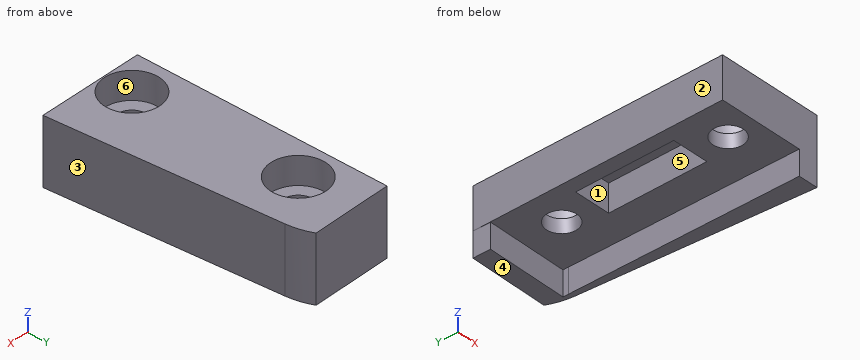
```python
from build123d import *

# Parameters (mm, degrees)
BOSS_EXTRUDE1_DEPTH = 1.8
SKETCH3_R           = 1.1
BOSS_EXTRUDE2_DEPTH = 3
SKETCH4_W           = 2.663520563
SKETCH4_H           = 7.169309516
CUT_EXTRUDE1_DEPTH  = 2
SKETCH5_R           = 2
CUT_EXTRUDE2_DEPTH  = 2


with BuildPart() as part:
    # Sketch1 → Boss-Extrude1 (new body)
    with BuildSketch(Plane(origin=(0, 0, 0), x_dir=(0, 1, 0), z_dir=(0, 0, 1))):
        with BuildLine():
            Line((6.830014349, -2.344806069), (-9.690684049, -3.631823148))
            Line((-9.690684049, -3.631823148), (-9.690684049, -2.205416312))
            Line((-9.690684049, -2.205416312), (6.947514193, -1.975901922))
            Line((6.947514193, -1.975901922), (7.350857331, -1.970338035))
            Line((7.350857331, -1.970338035), (7.269057374, 3.9595904))
            Line((7.269057374, 3.9595904), (8.531793523, 3.982646507))
            Line((8.531793523, 3.982646507), (8.638213972, -1.845785322))
            ThreePointArc((8.638213972, -1.845785322), (7.758081535, -2.182141378), (6.830014349, -2.344806069))
        make_face()
    extrude(amount=BOSS_EXTRUDE1_DEPTH)

    # Sketch3 → Boss-Extrude2 (add)
    with BuildSketch(Plane.XY.offset(1.8)):
        with BuildLine():
            Line((-3.982646507, 8.531793523), (-3.982646507, -9.690684049))
            Line((-3.982646507, -9.690684049), (3.631823148, -9.690684049))
            Line((3.631823148, -9.690684049), (2.344806069, 6.830014349))
            ThreePointArc((2.344806069, 6.830014349), (2.182141378, 7.758081535), (1.845785322, 8.638213972))
            Line((1.845785322, 8.638213972), (-3.982646507, 8.531793523))
        make_face()
        with Locations((-1.223821134, -7.594621825)):
            Circle(SKETCH3_R, mode=Mode.SUBTRACT)
        with Locations((-1.389338495, 4.404236621)):
            Circle(SKETCH3_R, mode=Mode.SUBTRACT)
    extrude(amount=BOSS_EXTRUDE2_DEPTH)

    # Sketch4 → Cut-Extrude1 (cut)
    with BuildSketch(Plane(origin=(0, 0, 1.8), x_dir=(1, 0, 0), z_dir=(0, 0, -1))):
        with Locations((-1.621806935, 1.615257833)):
            Rectangle(SKETCH4_W, SKETCH4_H)
    extrude(amount=-CUT_EXTRUDE1_DEPTH, mode=Mode.SUBTRACT)

    # Sketch5 → Cut-Extrude2 (cut)
    with BuildSketch(Plane.XY.offset(4.8)):
        with Locations((-1.389338495, 4.404236621)):
            Circle(SKETCH5_R)
        with Locations((-1.223821134, -7.594621825)):
            Circle(SKETCH5_R)
    extrude(amount=-CUT_EXTRUDE2_DEPTH, mode=Mode.SUBTRACT)


solid = part.part
```
Can you work these out from the model? Positions are in its coordinate system, mm. Face numbers are marked on the shaded views. A direction names the side the tool comes from. Give positions to 0.01 mm unless a question says otherwise; leave off trailing zeros. Loops run counter-clockwise (first coordinate to the right, second up) from the corner with the lowest first, then second, coordinate; pieces in that order, holes last. Notation, with made-up numbers: M 1.25,62 L 14.25,62 A24 cw 14.25,83 Z; hole C -7,51.25 d7. An arc over 180 degrees is marked long. Answer in a Markdown table with one row per item.
1. Which directions (+Z, -Z, +X, -X, +Y, -Y) give clear straight access to the entire face, cutting with the end or side of a thin tool? Please do the marked faces 4, 5 and 6.
Taken from the geometry:
| item | result |
|---|---|
| face 4 | -Z, +X, -X, +Y, -Y |
| face 5 | -Z |
| face 6 | +Z |
2. Thinking about a two-plate mould opening in X: for the marked faces 1, 2 and 3, which applies, released by +X, released by -X, zero draft, split by the parting line, or undercut?
Taken from the geometry:
| item | result |
|---|---|
| face 1 | undercut |
| face 2 | released by -X |
| face 3 | released by +X |
3. Suppose I cut it at A-A on z = 2.15. Write out the boundary of the cut face in (x, y), plus the area to 3 significant figures.
Taken from the geometry:
| item | result |
|---|---|
| outline | M -3.98,-9.69 L 3.63,-9.69 L 2.34,6.83 A4.93 ccw 1.85,8.64 L -3.98,8.53 Z; hole M -2.95,-5.2 L -0.29,-5.2 L -0.29,1.97 L -2.95,1.97 Z; hole C -1.39,4.4 d2.2; hole C -1.22,-7.59 d2.2 |
| area | 99.3 mm² |
4. For pin 1 Ø1.6 at (x, z) = (-1.5, 3) entering from +Y; pin 2 Ø1.2 at (x, y) = (-1.5, 5) entering from +Z; pin 3 Ø2 at (x, y) = (-2, -0.5) entering from -Z, each with a flat end and sliding along its axis, tell me the tip position at first contact or that it passes through.
Taken from the geometry:
| item | result |
|---|---|
| pin 1 | stops at y = 8.59 |
| pin 2 | stops at z = 2.8 |
| pin 3 | stops at z = 1.8 |
5. If I drill on line 1 along X through (y, z) = (1, 2.95); line 2 along Y through (x, z) = (-1.5, 2.2); line 3 along Y through (x, z) = (-1, 1.9), over which ranges is the centre line in solid material (lowest first)?
Taken from the geometry:
| item | result |
|---|---|
| line 1 | x = -3.98 to -2.95, -0.29 to 2.8 |
| line 2 | y = -9.69 to -8.66, -6.53 to -5.2, 1.97 to 3.31, 5.5 to 8.58 |
| line 3 | y = -9.69 to -8.67, -6.52 to -5.2, 1.97 to 3.38, 5.43 to 8.59 |
6. Suppose I cut it at C-C on z = 1.25. Write out the boundary of the cut face in (x, y), plus the area to 3 significant figures.
Taken from the geometry:
| item | result |
|---|---|
| outline | M -3.98,8.53 L -3.96,7.27 L 1.97,7.35 L 2.21,-9.69 L 3.63,-9.69 L 2.34,6.83 A4.93 ccw 1.85,8.64 Z |
| area | 22.7 mm² |
7. Suppose I cut it at D-D on z = 4.1. Write out the boundary of the cut face in (x, y).
Taken from the geometry:
| item | result |
|---|---|
| outline | M -3.98,-9.69 L 3.63,-9.69 L 2.34,6.83 A4.93 ccw 1.85,8.64 L -3.98,8.53 Z; hole C -1.39,4.4 d4; hole C -1.22,-7.59 d4 |
8. Suppose I cut it at B-B on y = 3.75. Write out the boundary of the cut face in (x, z).
Taken from the geometry:
| item | result |
|---|---|
| outline | M -3.98,1.8 L -2.27,1.8 L -2.27,2.8 L -3.28,2.8 L -3.28,4.8 L -3.98,4.8 Z; M -0.51,1.8 L 2.02,1.8 L 2.02,0 L 2.58,0 L 2.58,4.8 L 0.5,4.8 L 0.5,2.8 L -0.51,2.8 Z |
